Autodesk Inventor part; units mm, degrees
ref_plane "YZ Plane" through (0, 0, 0) normal (1, 0, 0) x (0, 1, 0)
ref_plane "XZ Plane" through (0, 0, 0) normal (0, 1, 0) x (-1, 0, 0)
ref_plane "XY Plane" through (0, 0, 0) normal (0, 0, 1) x (1, 0, 0)
sketch "Sketch1" plane through (0, 0, 0) normal (0, 0, 1) x (1, 0, 0)
  line L0 (0, 0) -> (0, 44.45)
  line L1 (0, 44.45) -> (12.7, 44.45)
  line L2 (0, 0) -> (76.2, 0)
  line L3 (76.2, 0) -> (76.2, 12.7)
  line L4 (76.2, 12.7) -> (50.8, 12.7)
  line L5 (44.45, 19.05) -> (44.45, 44.45)
  line L6 (44.45, 44.45) -> (31.75, 44.45)
  line L7 (31.75, 44.45) -> (31.75, 19.05)
  line L8 (12.7, 44.45) -> (12.7, 19.05)
  line L9 (12.7, 19.05) -> (31.75, 19.05)
  arc A0 (44.45, 19.05) -> (50.8, 12.7) centre (50.8, 19.05) ccw
  point P0 (44.45, 12.7)
  dimension "d0" = 44.45
  dimension "d1" = 12.7
  dimension "d2" = 76.2
  dimension "d3" = 12.7
  dimension "d4" = 31.75
  dimension "d5" = 31.75
  dimension "d6" = 12.7
  dimension "d7" = 25.4
  dimension "d8" = 25.4
  dimension "d9" = 19.05
  dimension "d26" = 6.35
extrude "Base" add sketch "Sketch1" along normal mid plane 50.8
sketch "Sketch2" plane through (0, 0, 25.4) normal (0, -1, 0) x (1, 0, 0)
  line L0 (76.2, -50.8) -> (76.2, 0)
  circle A0 centre (76.2, -25.4) radius 25.4
  point P0 (0, -25.4)
  point P1 (76.2, 0)
extrude "Circle_EXT" add sketch "Sketch2" against normal up to surface (12.7 mm away) contours L0 A0 picked at (83.8282, -21.7265)
sketch "Sketch3" plane through (44.45, 12.7, 25.4) normal (0, 1, 0) x (1, 0, 0)
  point P0 (-44.45, 25.4)
  point P1 (29.7441, 25.1789)
hole "Hole1" at (74.1941, 12.7, 0.2211) direction (0, -1, 0) diameter 19.05 end through all
sketch "Sketch4" plane through (44.45, 12.7, 25.4) normal (1, 0, 0) x (0, 0, -1)
  line L0 (0, 31.75) -> (0, 6.35)
  line L1 (0, 31.75) -> (50.8, 31.75)
  line L2 (12.7, 31.75) -> (12.7, 12.7)
  line L3 (12.7, 12.7) -> (38.1, 12.7)
  line L4 (38.1, 12.7) -> (38.1, 31.75)
  point P0 (25.4, -12.7)
  dimension "d22" = 19.05
  dimension "d23" = 25.4
extrude "RECT_CUT" cut sketch "Sketch4" against normal through all
properties part number "Saddle Bracket" material "Iron, Cast"
Build history of the part. All positions in model axes, mm. A direction names the side the tool comes from. Round coordinates to 2 decimals unless told otherwise and drop trailing zeros. Order: outer loops, then holes, each group sorted by start corner. A loop starts at its lowest first (then second) coordinate and runs counter-clockwise, first axis right, second up. Notation, with made-up numbers: M 36.25,42.5 L 66.25,42.5 A15 cw 66.25,65.5 Z; hole C 48.5,20 d2. An arc over 180 degrees is marked long. Use CSV: the item, a comma, the result in double quotes. Start each with the question number.
(1) Cut at C-C on y = 7. List the corners of the cut face in (x, z) (3 decimals), then the cut area to 3 significant figures.
(2) Cut at D-D on x = 72.5. List the corners of the cut face in (y, z), then the cut area to 3 significant figures.
(3) Tool access for faces 5 (the face through (44.45, 23, 0)), 6 (the face through (38, 35, 12.7)), 7 (the face through (22, 19.05, 0)): list every direction of +Z, -Z, +X, -X, +Y, -Y with a clear straight run to the whole face (end or side of a thin tool).
(4) Mould opens along Z. For faces 1 (the face through (29, 18, 25.4)), 2 (the face through (67.76, 6.26, -6.8)), 3 (the face through (12.7, 23, 0)), 4 (the face through (101.594, 6.261, -0.559)) say: +Z half, -Z half, draft (parallel to the pull), parting line (faces both ways), or undercut.
(5) Flat gauge pins, fed straight in: P1, Ø6, axis at x = 84, z = 13, coming from the +Y side; P2, Ø5.5, axis at x = 25, z = 1, coming from the +Y side; P3, Ø4, axis at x = 38.5, z = 0, coming from the +Y side. Where does each tip first touch, or does it go through?
(6) Drill centre lines: probe 1 along Z at (x, y) = (33.5, 27); probe 2 along X at (y, z) = (23.5, -19); probe 3 along Y at (x, z) = (51.5, 13). Where is each one in solid material? Low to high.
(7) Cut at A-A on x = 40.5. List the corners of the cut face in (y, z).
(8) Cut at B-B on z = -5. List the corners of the cut face in (x, y).
Findings:
1,outline,"M 0,-25.4 L 76.2,-25.4 A25.4 ccw 76.2,25.4 L 0,25.4 Z; hole C 74.194,0.221 d19.05"
1,area,"4,600 mm^2"
2,outline,"M 0,-25.4 L 12.7,-25.4 L 12.7,-9.15 L 0,-9.15 Z; M 0,9.59 L 12.7,9.59 L 12.7,25.4 L 0,25.4 Z"
2,area,"407 mm^2"
3,face 5,"+Z, -Z, +X, +Y"
3,face 6,"+X, -X, +Y"
3,face 7,"+Z, -Z, +Y"
4,face 1,"+Z half"
4,face 2,"undercut"
4,face 3,"draft"
4,face 4,"parting line"
5,P1,"stops at y = 12.7"
5,P2,"stops at y = 19.05"
5,P3,"stops at y = 25.4"
6,probe 1,"z = -25.4 to -12.7, 12.7 to 25.4"
6,probe 2,"x = 0 to 12.7, 31.75 to 44.45"
6,probe 3,"y = 0 to 12.7"
7,outline,"M 0,-25.4 L 44.45,-25.4 L 44.45,-12.7 L 25.4,-12.7 L 25.4,12.7 L 44.45,12.7 L 44.45,25.4 L 0,25.4 Z"
8,outline,"M 0,0 L 66.23,0 L 66.23,12.7 L 50.8,12.7 A6.35 cw 44.45,19.05 L 44.45,25.4 L 31.75,25.4 L 31.75,19.05 L 12.7,19.05 L 12.7,25.4 L 0,25.4 Z; M 82.16,0 L 101.1,0 L 101.1,12.7 L 82.16,12.7 Z"
